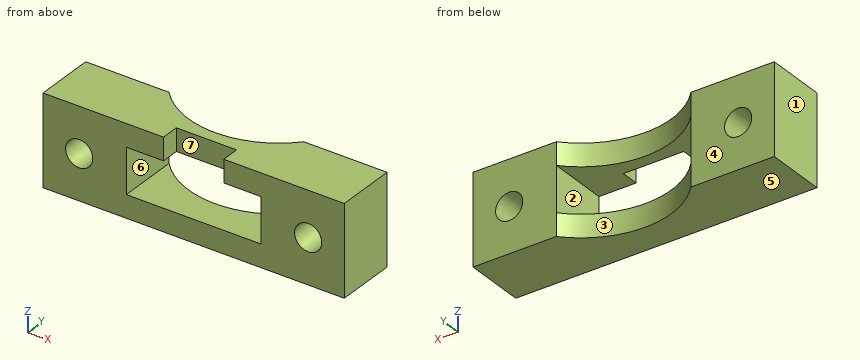
```python
from build123d import *

# Parameters (mm, degrees)
BOSS_EXTRUDE1_DEPTH = 15
CUT_EXTRUDE1_REACH  = 32.822
SKETCH3_W           = 22.360679774
SKETCH3_H           = 7.5
CUT_EXTRUDE2_REACH  = 31.58
SKETCH2_W           = 10
SKETCH2_H           = 3
CUT_EXTRUDE3_REACH  = 32.822
SKETCH4_R           = 2.25
SHELL2_START        = 1
SHELL2_OUTLINE_W    = 11.819660113
SHELL2_OUTLINE_H    = 8
SHELL2_DEPTH        = 3.2499999
SHELL2_START_2      = 10.7500001
SHELL2_2_OUTLINE_W  = 11.819660113
SHELL2_2_OUTLINE_H  = 8
SHELL2_2_DEPTH      = 3.2499999
SHELL2_3_DEPTH      = 1.75
SHELL2_START_3      = 12.25
SHELL2_4_DEPTH      = 1.75
SHELL2_START_4      = -4
SHELL2_5_DEPTH      = 8


with BuildPart() as part:
    # Sketch1 → Boss-Extrude1 (new body)
    with BuildSketch(Plane.XY):
        with BuildLine():
            Line((-25, 5), (-11.180339887, 5))
            ThreePointArc((-11.180339887, 5), (0, 0), (11.180339887, 5))
            Line((11.180339887, 5), (25, 5))
            Line((25, 5), (25, -5))
            Line((25, -5), (-25, -5))
            Line((-25, -5), (-25, 5))
        make_face()
    extrude(amount=BOSS_EXTRUDE1_DEPTH)

    # Sketch3 → Cut-Extrude1 (cut, up to next)
    with BuildSketch(Plane(origin=(0, 5, 0), x_dir=(1, 0, 0), z_dir=(0, 1, 0)), mode=Mode.PRIVATE) as cut_extrude1_sk1:
        with Locations((0, -7.5)):
            Rectangle(SKETCH3_W, SKETCH3_H)
    cut_extrude1_tool1 = extrude(cut_extrude1_sk1.sketch, amount=-CUT_EXTRUDE1_REACH, mode=Mode.PRIVATE) & part.part
    add(cut_extrude1_tool1.solids().sort_by_distance((0, 5, 7.5))[0], mode=Mode.SUBTRACT)

    # Sketch2 → Cut-Extrude2 (cut, up to next)
    with BuildSketch(Plane.XY.offset(15), mode=Mode.PRIVATE) as cut_extrude2_sk1:
        with Locations((0, -3.5)):
            Rectangle(SKETCH2_W, SKETCH2_H)
    cut_extrude2_tool1 = extrude(cut_extrude2_sk1.sketch, amount=-CUT_EXTRUDE2_REACH, mode=Mode.PRIVATE) & part.part
    add(cut_extrude2_tool1.solids().sort_by_distance((0, -3.5, 15))[0], mode=Mode.SUBTRACT)

    # Sketch4 → Cut-Extrude3 (cut, up to next)
    with BuildSketch(Plane(origin=(0, 5, 0), x_dir=(1, 0, 0), z_dir=(0, 1, 0)), mode=Mode.PRIVATE) as cut_extrude3_sk1:
        with Locations(Location((-19, -7.5, 0), (0, 0, 270))):
            Circle(SKETCH4_R)
    cut_extrude3_tool1 = extrude(cut_extrude3_sk1.sketch, amount=-CUT_EXTRUDE3_REACH, mode=Mode.PRIVATE) & part.part
    # Sketch4 → Cut-Extrude3 (cut, up to next)
    with BuildSketch(Plane(origin=(0, 5, 0), x_dir=(1, 0, 0), z_dir=(0, 1, 0)), mode=Mode.PRIVATE) as cut_extrude3_sk2:
        with Locations(Location((19, -7.5, 0), (0, 0, 270))):
            Circle(SKETCH4_R)
    cut_extrude3_tool2 = extrude(cut_extrude3_sk2.sketch, amount=-CUT_EXTRUDE3_REACH, mode=Mode.PRIVATE) & part.part
    add(cut_extrude3_tool1.solids().sort_by_distance((-19, 5, 7.5))[0], mode=Mode.SUBTRACT)
    add(cut_extrude3_tool2.solids().sort_by_distance((19, 5, 7.5))[0], mode=Mode.SUBTRACT)

    # Shell2: read off the stored shape, not the designer's step
    # Shell2 outline → Shell2 (cut)
    with BuildSketch(Plane.XY.offset(SHELL2_START)):
        with Locations((18.090169944, 0)):
            Rectangle(SHELL2_OUTLINE_W, SHELL2_OUTLINE_H)
        with Locations((-18.090169944, 0)):
            Rectangle(SHELL2_OUTLINE_W, SHELL2_OUTLINE_H)
    extrude(amount=SHELL2_DEPTH, mode=Mode.SUBTRACT)

    # Shell2 2 outline → Shell2 2 (cut)
    with BuildSketch(Plane.XY.offset(SHELL2_START_2)):
        with Locations((18.090169944, 0)):
            Rectangle(SHELL2_2_OUTLINE_W, SHELL2_2_OUTLINE_H)
        with Locations((-18.090169944, 0)):
            Rectangle(SHELL2_2_OUTLINE_W, SHELL2_2_OUTLINE_H)
    extrude(amount=SHELL2_2_DEPTH, mode=Mode.SUBTRACT)

    # Shell2 3 outline → Shell2 3 (cut)
    with BuildSketch(Plane.XY.offset(SHELL2_START)):
        with BuildLine():
            Line((12.180339887, 4), (11.618950039, 4))
            ThreePointArc((11.618950039, 4), (0, -1), (-11.618950039, 4))
            Line((-11.618950039, 4), (-12.180339887, 4))
            Line((-12.180339887, 4), (-12.180339887, -4))
            Line((-12.180339887, -4), (12.180339887, -4))
            Line((12.180339887, -4), (12.180339887, 4))
        make_face()
    extrude(amount=SHELL2_3_DEPTH, mode=Mode.SUBTRACT)

    # Shell2 4 outline → Shell2 4 (cut)
    with BuildSketch(Plane.XY.offset(SHELL2_START_3)):
        with BuildLine():
            Line((12.180339887, 4), (11.618950039, 4))
            ThreePointArc((11.618950039, 4), (6.324555321, 0.303061543), (0, -1))
            Line((0, -1), (6, -1))
            Line((6, -1), (6, -4))
            Line((6, -4), (12.180339887, -4))
            Line((12.180339887, -4), (12.180339887, 4))
        make_face()
        with BuildLine():
            Line((-6, -1), (0, -1))
            ThreePointArc((0, -1), (-6.324555321, 0.303061543), (-11.618950039, 4))
            Line((-11.618950039, 4), (-12.180339887, 4))
            Line((-12.180339887, 4), (-12.180339887, -4))
            Line((-12.180339887, -4), (-6, -4))
            Line((-6, -4), (-6, -1))
        make_face()
    extrude(amount=SHELL2_4_DEPTH, mode=Mode.SUBTRACT)

    # Shell2 5 outline → Shell2 5 (cut)
    with BuildSketch(Plane(origin=(0, 0, 0), x_dir=(1, 0, 0), z_dir=(0, 1, 0)).offset(SHELL2_START_4)):
        with BuildLine():
            Line((24, -10.7500001), (24, -4.2499999))
            Line((24, -4.2499999), (19, -4.25))
            ThreePointArc((19, -4.25), (22.25, -7.5), (19, -10.75))
            Line((19, -10.75), (24, -10.7500001))
        make_face()
        with BuildLine():
            ThreePointArc((19, -10.75), (15.75, -7.5), (19, -4.25))
            Line((19, -4.25), (12.180339887, -4.2499999))
            Line((12.180339887, -4.2499999), (12.180339887, -10.7500001))
            Line((12.180339887, -10.7500001), (19, -10.75))
        make_face()
        with BuildLine():
            Line((-24, -4.2499999), (-24, -10.7500001))
            Line((-24, -10.7500001), (-19, -10.75))
            ThreePointArc((-19, -10.75), (-22.25, -7.5), (-19, -4.25))
            Line((-19, -4.25), (-24, -4.2499999))
        make_face()
        with BuildLine():
            ThreePointArc((-19, -4.25), (-15.75, -7.5), (-19, -10.75))
            Line((-19, -10.75), (-12.180339887, -10.7500001))
            Line((-12.180339887, -10.7500001), (-12.180339887, -4.2499999))
            Line((-12.180339887, -4.2499999), (-19, -4.25))
        make_face()
    extrude(amount=SHELL2_5_DEPTH, mode=Mode.SUBTRACT)


solid = part.part
```
Source: CAD feature listing. Evaluate the final solid. Frame: model axes, mm. Face numbers are marked on the shaded views. A direction names the side the tool comes from. Coordinates: 2 decimals unless noted, no trailing zeros. Order: outer loops, then holes, each group sorted by start corner. A loop starts at its lowest first (then second) coordinate and runs counter-clockwise, first axis right, second up. Notation, with made-up numbers: M 22.25,-20.75 L 35.25,-20.75 A16 ccw 35.25,7.25 Z; hole C 8,-17.75 d9. An arc over 180 degrees is marked long. Write each question's results on one line, items separated by ' | '. Start each with the question number.
1) Line query: line 1 (Z direction, x = -5, y = -1.75); line 2 (X direction, y = -1.5, z = 13.25); line 3 (Y direction, x = -17, z = 13.5). Output: solid intervals per line, ascending. Write a range as from..to.
2) Section query C-C (x = -19). Return the cut outline in (y, z).
3) Access query for the marked faces 5, 6 and 7. Directions: +Z, -Z, +X, -X, +Y, -Y. A direction counts if a zero-diameter tool reaches every point of the face in a straight line with its end or side. Return the directions, or none.
4) Section query B-B (y = -2.75). Return the cut outline in (x, z).
5) Contact query for flat-ended pins moving along their axis: pin 1 Ø4 at (x, y) = (-4.5, 0.5) entering from -Z; pin 2 Ø2.5 at (x, y) = (-1.5, 1.5) entering from +Z; pin 3 Ø1.9 at (x, z) = (2, 12.5) entering from +Y; pin 4 Ø3 at (x, z) = (7.5, 3) entering from +Y. Output: stop coordinate, or through.
6) Section query A-A (z = 7.5). Give the number of separate pieces and of enclosed holes in the cut face, plus the area to 3 significant figures.
7) Draft query along X for the marked faces 1, 2, 3 and 4. Return one class per face: released by +X, released by -X, zero draft, split by the parting line, or undercut.
Answers:
1) line 1: z = 0..1, 2.75..3.75, 11.25..15 | line 2: x = -25..-24, -6..6, 24..25 | line 3: y = -5..-4, 4..5
2) outline: M -5,0 L 5,0 L 5,5.25 L -5,5.25 Z; M -5,9.75 L 5,9.75 L 5,15 L -5,15 Z; hole M -4,1 L 4,1 L 4,4.25 L -4,4.25 Z; hole M -4,10.75 L 4,10.75 L 4,14 L -4,14 Z
3) face 5: -Z, +X, -X, +Y, -Y | face 6: +Y, -Y | face 7: +Z, -Y
4) outline: M -25,0 L 25,0 L 25,15 L 5,15 L 5,11.25 L 11.18,11.25 L 11.18,3.75 L -11.18,3.75 L -11.18,11.25 L -5,11.25 L -5,15 L -25,15 Z; C -19,7.5 d6.5; C 19,7.5 d6.5; hole M -24,1 L 24,1 L 24,14 L 6,14 L 6,12.25 L 12.18,12.25 L 12.18,2.75 L -12.18,2.75 L -12.18,12.25 L -6,12.25 L -6,14 L -24,14 Z; hole C -19,7.5 d4.5; hole C 19,7.5 d4.5
5) pin 1: stops at z = 0 | pin 2: passes through | pin 3: stops at y = 0.29 | pin 4: stops at y = 3
6) separate pieces: 4 | enclosed holes: 4 | area: 101 mm^2
7) face 1: released by -X | face 2: undercut | face 3: undercut | face 4: zero draft
